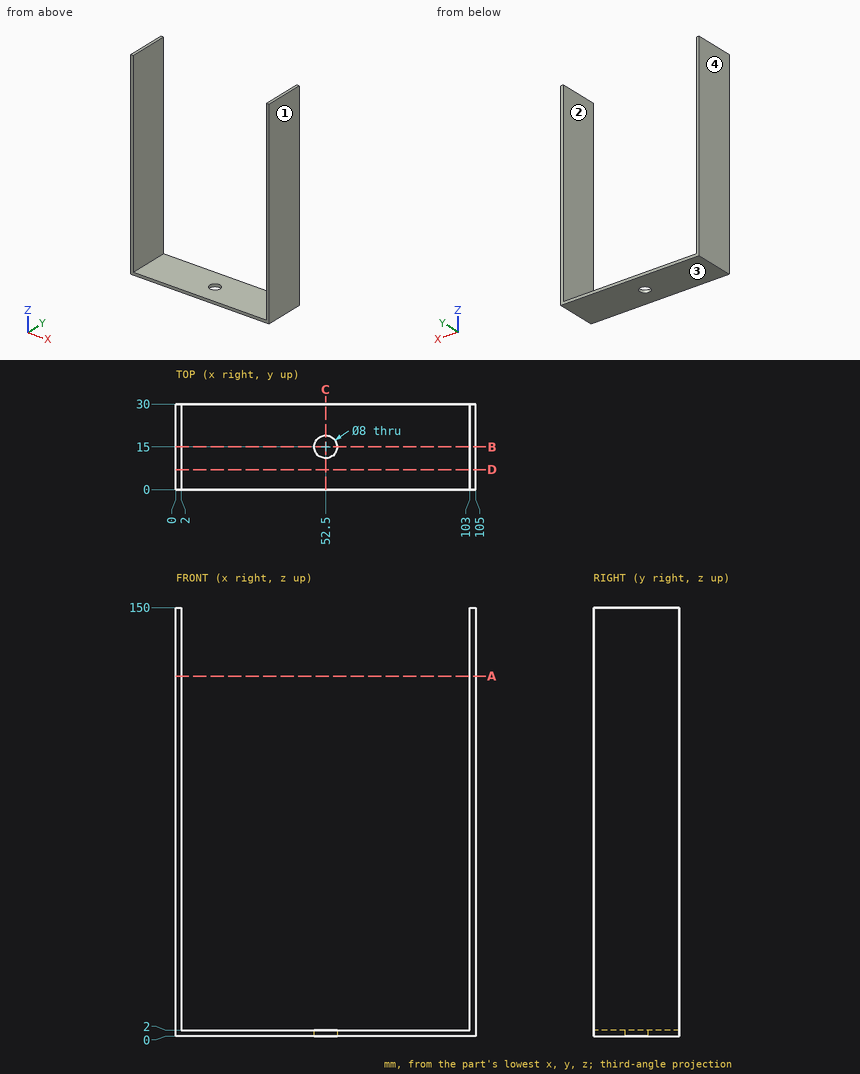
Print and shaded views of the part. All mm, measured from the part's lowest x, y and z. Coordinates: 2 decimals unless noted, no trailing zeros. Loops run counter-clockwise (first coordinate to the right, second up) from the corner with the lowest first, then second, coordinate; pieces in that order, holes last. Notation, with made-up numbers: M 69,86 L 86,86 A28 ccw 86,115 Z; hole C 16.25,54.5 d11. An arc over 180 degrees is marked long. Use a Markdown table: item, result. Add a question column.
Q1. Mould opens along X. For the marked faces 1, 2, 3 and 4 say: +X half, -X half, draft (parallel to the pull), parting line (faces both ways), or undercut.
Q2. Cut at C-C (x = 52.5). Write the cut outline in (y, z), and give its area (3 significant figures).
Q3. Cut at A-A (z = 126). Write the cut outline in (x, y).
Q4. Cut at D-D (y = 7). Write the cut outline in (x, z).
Q5. Probe L1, parallel to Y at x = 52, z = 1; L2, parallel to X at y = 25.5, z = 98.5; L3, parallel to Z at x = 66.5, y = 18.75. List the from-to ranges inside material, lowest first.
Q6. Pin check, flat tips, straight feed: P1, Ø8, axis at x = 75, y = 24.5, coming from the -Z side; P2, Ø10, axis at x = 16, y = 15, coming from the +Z side. Stop position of each tip, or through.
Q7. Cut at B-B (y = 15). Write the cut outline in (x, z), and give its area (3 significant figures).
Worked out:
| question | item | result |
|---|---|---|
| 1 | face 1 | +X half |
| 1 | face 2 | undercut |
| 1 | face 3 | draft |
| 1 | face 4 | -X half |
| 2 | outline | M 0,0 L 11,0 L 11,2 L 0,2 Z; M 19,0 L 30,0 L 30,2 L 19,2 Z |
| 2 | area | 44.0 mm2 |
| 3 | outline | M 0,0 L 2,0 L 2,30 L 0,30 Z; M 103,0 L 105,0 L 105,30 L 103,30 Z |
| 4 | outline | M 0,0 L 105,0 L 105,150 L 103,150 L 103,2 L 2,2 L 2,150 L 0,150 Z |
| 5 | L1 | y = 0 to 11.03, 18.97 to 30 |
| 5 | L2 | x = 0 to 2, 103 to 105 |
| 5 | L3 | z = 0 to 2 |
| 6 | P1 | stops at z = 0 |
| 6 | P2 | stops at z = 2 |
| 7 | outline | M 0,0 L 48.5,0 L 48.5,2 L 2,2 L 2,150 L 0,150 Z; M 56.5,0 L 105,0 L 105,150 L 103,150 L 103,2 L 56.5,2 Z |
| 7 | area | 786 mm2 |
